Can you work these out from the drawing? Everything is in mm from the part's minimum corner. A direction names the side the tool comes from. Give positions to 0.01 mm unless a question says otherwise; leave off trailing zeros. Order: outer loops, then holes, each group sorted by start corner. A loop starts at its lowest first (then second) coordinate and runs counter-clockwise, first axis right, second up. Notation, with made-up numbers: M 38,79 L 60,79 A18 cw 60,114 Z; hole C 20.5,69 d8. An arc over 180 degrees is marked long. Use a Markdown table: item, result. Add a question column.
Item 1: Suppose I cut it at A-A on x = 35. Write out the boundary of the cut face in (y, z).
Item 2: Suppose I cut it at B-B on z = 36. Write out the boundary of the cut face in (x, y), plus the area to 3 significant figures.
Item 3: Suppose I cut it at C-C on z = 55.5. Write out the boundary of the cut face in (x, y), plus the area to 3 significant figures.
Item 4: I'm going to push flat-ended pins straight in: pin 1 Ø15 at (y, z) = (69.5, 26) entering from -X; pin 2 Ø4 at (y, z) = (12, 87) entering from -X. Where does each tip first touch, or does it pass through?
Item 5: If I drill on L1, parallel to Z at x = 35, y = 42; L2, parallel to X at y = 96, z = 43, over which ranges is the centre line in solid material (lowest first)? Write a range as from..to.
Item 6: For the marked faces 1, 2 and 3, which set-ups out of +Z, -Z, +X, -X, +Y, -Y let a thin tool reach every point of the face, with its end or its side?
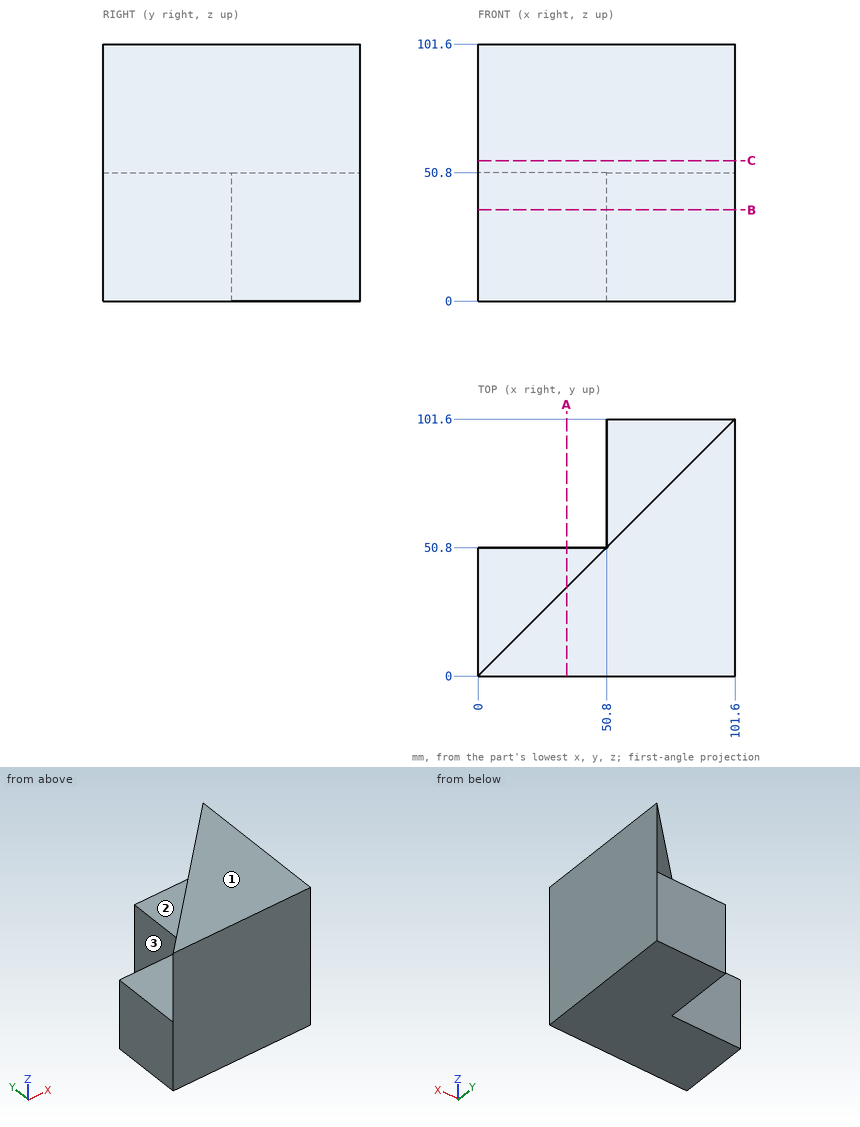
Findings below:
| question | item | result |
|---|---|---|
| 1 | outline | M 0,0 L 50.8,0 L 50.8,50.8 L 35,50.8 L 35,101.6 L 0,101.6 Z |
| 2 | outline | M 0,0 L 101.6,0 L 101.6,101.6 L 50.8,101.6 L 50.8,50.8 L 0,50.8 Z |
| 2 | area | 7,740 mm^2 |
| 3 | outline | M 0,0 L 101.6,0 L 101.6,101.6 Z |
| 3 | area | 5,160 mm^2 |
| 4 | pin 1 | stops at x = 50.8 |
| 4 | pin 2 | stops at x = 10 |
| 5 | L1 | z = 0..50.8 |
| 5 | L2 | x = 50.8..101.6 |
| 6 | face 1 | +Z, +X, -X, +Y, -Y |
| 6 | face 2 | +Z, -X, +Y |
| 6 | face 3 | +Z, -Z, -X, +Y |
